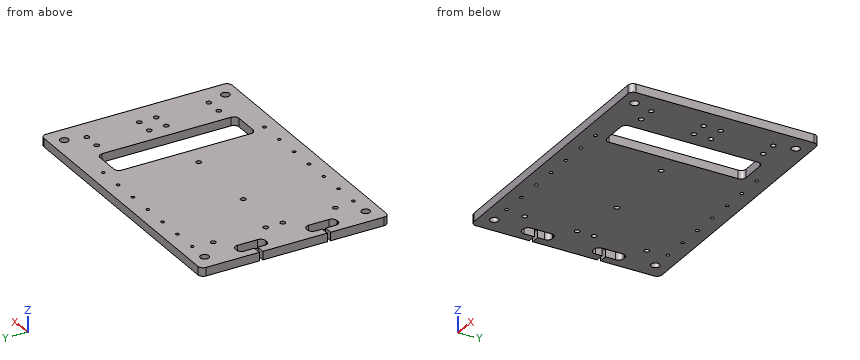
from build123d import *

# Parameters (mm, degrees)
SKETCH_1_W          = 162
SKETCH_1_H          = 111
EXTRUDE_1_DEPTH     = 5
CUT_EXTRUDE_1_REACH = 198.443
SKETCH_2_W          = 20
SKETCH_2_H          = 82
SKETCH_3_R          = 1.5
SKETCH_3_R_2        = 1
SKETCH_3_R_3        = 2.5
SKETCH_3_W          = 7
SKETCH_3_H          = 60
CUT_EXTRUDE_2_DEPTH = 5
FILLET_1_R          = 3
CUT_EXTRUDE_3_REACH = 198.443
SKETCH_4_R          = 1
SKETCH2_W           = 7
SKETCH2_H           = 24
BOSS_EXTRUDE2_DEPTH = 5
SKETCH3_W           = 5
SKETCH3_H           = 2
CUT_EXTRUDE1_DEPTH  = 197.443376065
FILLET1_R           = 3


with BuildPart() as part:
    # 草图1 → 凸台-拉伸1 (new body)
    with BuildSketch(Plane.XY):
        with Locations((81, -55.5)):
            Rectangle(SKETCH_1_W, SKETCH_1_H)
    extrude(amount=EXTRUDE_1_DEPTH)

    # 草图2 → 切除-拉伸1 (cut, up to next)
    with BuildSketch(Plane(origin=(0, 0, 0), x_dir=(-1, 0, 0), z_dir=(0, 0, -1)), mode=Mode.PRIVATE) as cut_extrude_1_sk1:
        with Locations((-120, -55.5)):
            Rectangle(SKETCH_2_W, SKETCH_2_H)
    cut_extrude_1_tool1 = extrude(cut_extrude_1_sk1.sketch, amount=-CUT_EXTRUDE_1_REACH, mode=Mode.PRIVATE) & part.part
    add(cut_extrude_1_tool1.solids().sort_by_distance((120, -55.5, 0))[0], mode=Mode.SUBTRACT)

    # 草图3 → 切除-拉伸2 (cut)
    with BuildSketch(Plane.XY.offset(5)):
        with Locations((149, -60.5)):
            Circle(SKETCH_3_R)
        with Locations((139, -60.5)):
            Circle(SKETCH_3_R)
        with Locations((149, -91.5)):
            Circle(SKETCH_3_R)
        with Locations((139, -91.5)):
            Circle(SKETCH_3_R)
        with Locations((149, -50.5)):
            Circle(SKETCH_3_R)
        with Locations((139, -50.5)):
            Circle(SKETCH_3_R)
        with Locations((22.5, -103)):
            Circle(SKETCH_3_R_2)
        with Locations((22.5, -8)):
            Circle(SKETCH_3_R_2)
        with Locations((21, -60.5)):
            Circle(SKETCH_3_R)
        with Locations((21, -91.5)):
            Circle(SKETCH_3_R)
        with Locations((21, -50.5)):
            Circle(SKETCH_3_R)
        with Locations((21, -19.5)):
            Circle(SKETCH_3_R)
        with Locations((10, -8)):
            Circle(SKETCH_3_R_3)
        with Locations((152, -8)):
            Circle(SKETCH_3_R_3)
        with Locations((152, -103)):
            Circle(SKETCH_3_R_3)
        with Locations((10, -103)):
            Circle(SKETCH_3_R_3)
        with Locations((37.5, -103)):
            Circle(SKETCH_3_R_2)
        with Locations((52.5, -103)):
            Circle(SKETCH_3_R_2)
        with Locations((67.5, -103)):
            Circle(SKETCH_3_R_2)
        with Locations((82.5, -103)):
            Circle(SKETCH_3_R_2)
        with Locations((97.5, -103)):
            Circle(SKETCH_3_R_2)
        with Locations((37.5, -8)):
            Circle(SKETCH_3_R_2)
        with Locations((52.5, -8)):
            Circle(SKETCH_3_R_2)
        with Locations((67.5, -8)):
            Circle(SKETCH_3_R_2)
        with Locations((82.5, -8)):
            Circle(SKETCH_3_R_2)
        with Locations((97.5, -8)):
            Circle(SKETCH_3_R_2)
        with Locations((112.5, -8)):
            Circle(SKETCH_3_R_2)
        with Locations((139, -19.5)):
            Circle(SKETCH_3_R)
        with Locations((149, -19.5)):
            Circle(SKETCH_3_R)
        with Locations((112.5, -103)):
            Circle(SKETCH_3_R_2)
        with Locations((52.5, -55.5)):
            Circle(SKETCH_3_R)
        with Locations((97.5, -55.5)):
            Circle(SKETCH_3_R)
        with Locations((8.5, -55.5)):
            Rectangle(SKETCH_3_W, SKETCH_3_H)
    extrude(amount=-CUT_EXTRUDE_2_DEPTH, mode=Mode.SUBTRACT)

    # 圆角1
    fillet_1_edges = [part.edges().sort_by_distance(p)[0] for p in [
        (5, -25.5, 2.5),
        (12, -25.5, 2.5),
        (12, -85.5, 2.5),
        (5, -85.5, 2.5),
        (110, -96.5, 2.5),
        (130, -96.5, 2.5),
        (130, -14.5, 2.5),
        (110, -14.5, 2.5),
        (0, 0, 2.5),
        (162, 0, 2.5),
        (162, -111, 2.5),
        (0, -111, 2.5),
    ]]
    fillet(fillet_1_edges, radius=FILLET_1_R)

    # 草图4 → 切除-拉伸3 (cut, up to next)
    with BuildSketch(Plane.ZY, mode=Mode.PRIVATE) as cut_extrude_3_sk1:
        with Locations(Location((2.5, -35.5, 0), (0, 0, 270))):
            Circle(SKETCH_4_R)
    cut_extrude_3_tool1 = extrude(cut_extrude_3_sk1.sketch, amount=-CUT_EXTRUDE_3_REACH, mode=Mode.PRIVATE) & part.part
    # 草图4 → 切除-拉伸3 (cut, up to next)
    with BuildSketch(Plane.ZY, mode=Mode.PRIVATE) as cut_extrude_3_sk2:
        with Locations(Location((2.5, -75.5, 0), (0, 0, 270))):
            Circle(SKETCH_4_R)
    cut_extrude_3_tool2 = extrude(cut_extrude_3_sk2.sketch, amount=-CUT_EXTRUDE_3_REACH, mode=Mode.PRIVATE) & part.part
    add(cut_extrude_3_tool1.solids().sort_by_distance((0, -35.5, 2.5))[0], mode=Mode.SUBTRACT)
    add(cut_extrude_3_tool2.solids().sort_by_distance((0, -75.5, 2.5))[0], mode=Mode.SUBTRACT)

    # Sketch2 → Boss-Extrude2 (add)
    with BuildSketch(Plane.XY):
        with Locations((8.5, -55.5)):
            Rectangle(SKETCH2_W, SKETCH2_H)
    extrude(amount=BOSS_EXTRUDE2_DEPTH)

    # Sketch3 → Cut-Extrude1 (cut, through all)
    with BuildSketch(Plane.XY.offset(5)):
        with Locations((2.5, -35.5)):
            Rectangle(SKETCH3_W, SKETCH3_H)
        with Locations((2.5, -75.5)):
            Rectangle(SKETCH3_W, SKETCH3_H)
    extrude(amount=-CUT_EXTRUDE1_DEPTH, mode=Mode.SUBTRACT)

    # Fillet1
    fillet1_edges = [part.edges().sort_by_distance(p)[0] for p in [
        (5, -67.5, 2.5),
        (12, -67.5, 2.5),
        (12, -43.5, 2.5),
        (5, -43.5, 2.5),
    ]]
    fillet(fillet1_edges, radius=FILLET1_R)


solid = part.part
Read the model definition and answer for the solid it produces. Units are mm, in the model's axes. Round coordinates to 2 decimals unless told otherwise and drop trailing zeros. Loops run counter-clockwise (first coordinate to the right, second up) from the corner with the lowest first, then second, coordinate; pieces in that order, holes last.
Q1. Section B-B on z = 1.15 is taken. Give the number of separate pieces and of enclosed holes in the cut face, and give its area (3 significant figures).
Q2. Consider probe 1 along X at (y, z) = (-91.5, 2.6); probe 2 along X at (y, z) = (-28.5, 0.45); probe 3 along Y at (x, z) = (117, 4.55). Determine where each line is inside the solid, lowest interval first.
Q3. Section A-A on x = 116 is taken. Write down the section's boundary in (y, z).
Output:
1. separate pieces: 1
1. enclosed holes: 33
1. area: 15,900 mm2
2. probe 1: x = 0 to 19.5, 22.5 to 110, 130 to 137.5, 140.5 to 147.5, 150.5 to 162
2. probe 2: x = 0 to 5, 12 to 110, 130 to 162
2. probe 3: y = -111 to -96.5, -14.5 to 0
3. outline: (-111, 0) - (-96.5, 0) - (-96.5, 5) - (-111, 5) - close; (-14.5, 0) - (0, 0) - (0, 5) - (-14.5, 5) - close
